```python
from build123d import *

# Parameters (mm, degrees)
SKETCH_1_R          = 3.25
EXTRUDE_1_DEPTH     = 28
SKETCH_3_R          = 4.25
CUT_EXTRUDE_1_DEPTH = 17


with BuildPart() as part:
    # 草图1 → 凸台-拉伸1 (new, symmetric)
    with BuildSketch(Plane.XY):
        with BuildLine():
            Line((-77.585786438, 0), (0, 0))
            Line((0, 0), (0, 8))
            Line((0, 8), (-17.995464086, 8))
            Line((-17.995464086, 8), (-30.499317942, 38.186973559))
            Line((-30.499317942, 38.186973559), (-17.774603256, 50.911688245))
            Line((-17.774603256, 50.911688245), (-23.431457505, 56.568542495))
            Line((-23.431457505, 56.568542495), (-78.292893219, 1.707106781))
            ThreePointArc((-78.292893219, 1.707106781), (-78.50966597, 0.617316568), (-77.585786438, 0))
        make_face()
        with Locations((-57.82689122, 9.184402377)):
            Circle(SKETCH_1_R, mode=Mode.SUBTRACT)
        Polygon((-67.928932188, 5), (-63.07447047, 5), (-64.496309389, 8.4326228), align=None, mode=Mode.SUBTRACT)
        with BuildLine():
            Line((-54.257468753, 5), (-20, 5))
            Line((-20, 5), (-34.038059223, 38.890872965))
            Line((-34.038059223, 38.890872965), (-58.261747684, 14.667184504))
            ThreePointArc((-58.261747684, 14.667184504), (-52.745553791, 11.289161255), (-54.257468753, 5))
        make_face(mode=Mode.SUBTRACT)
    extrude(amount=EXTRUDE_1_DEPTH, both=True)

    # 草图3 → 切除-拉伸1 (cut)
    with BuildSketch(Plane(origin=(0, 8, 0), x_dir=(1, 0, 0), z_dir=(0, 1, 0))):
        with Locations(Location((-10, -15, 0), (0, 0, 180))):
            Circle(SKETCH_3_R)
        with Locations(Location((-10, 15, 0), (0, 0, 270))):
            Circle(SKETCH_3_R)
    cut_extrude_1 = extrude(amount=-CUT_EXTRUDE_1_DEPTH, mode=Mode.SUBTRACT)

    # 镜向1: 切除-拉伸1 across plane
    add(cut_extrude_1.mirror(Plane(origin=(-11.715728753, 28.284271247, 0), x_dir=(0, 0, 1), z_dir=(-0.3826834323650881, 0.9238795325112875, 0))), mode=Mode.SUBTRACT)


solid = part.part
```
Design review of the part built by this model. Coordinates are the model's own, in mm. A direction names the side the tool comes from. Coordinates: 2 decimals unless noted, no trailing zeros. Order: outer loops, then holes, each group sorted by start corner. A loop starts at its lowest first (then second) coordinate and runs counter-clockwise, first axis right, second up. Notation, with made-up numbers: (60, 39) - (98, 39) arc R25 cw to (98, 73) - close; hole circle Ø11 at (8, -7.75). An arc over 180 degrees is marked (long way). Answer in a Markdown table with one row per item.
(1) Consider section C-C on y = 35. State the section outline as (x, z) points.
Checked values:
| item | result |
|---|---|
| outline | (-45, -28) - (-37.93, -28) - (-37.93, 28) - (-45, 28) - close; (-32.43, -28) - (-29.18, -28) - (-29.18, 28) - (-32.43, 28) - close |
(2) For faces 5 (the flat face through (0, 4, 0)), 6 (the flat face through (-63.775, 6.692, 0.392)), list the 3-axis set-ups (+Z, -Z, +X, -X, +Y, -Y) from which the entire face can be reached by the end or side of a thin tool; tool diameter is ignored.
Checked values:
| item | result |
|---|---|
| face 5 | +Z, -Z, +X, +Y, -Y |
| face 6 | +Z, -Z |
(3) The part is to be moulded in two halves that separate along Y. For faces 1 (the flat face through (-45.98, 26.95, 0.39)), 2 (the flat face through (-51.1, 22.1, -28)), 3 (the cylindrical face through (-78.516, 0.633, 0.392)), 4 (the flat face through (-50, 30, 0)), say which applies: released by +Y, released by -Y, zero draft, split by the parting line, or undercut.
Checked values:
| item | result |
|---|---|
| face 1 | undercut |
| face 2 | zero draft |
| face 3 | split by the parting line |
| face 4 | released by +Y |
(4) Clearance check with flat-ended pins moving along their axes: pin 1 (7.5 mm diameter, centred on x = -10, z = 15, fed in from +Y); pin 2 (2.5 mm diameter, centred on x = -65.5, z = 11.5, fed in from +Y); pin 3 (2 mm diameter, centred on x = -51.5, z = -15.5, fed in from +Y); pin 4 (3 mm diameter, centred on x = -47, z = 19, fed in from +Y). State where each tip first meets the part, or that it passes through.
Checked values:
| item | result |
|---|---|
| pin 1 | through |
| pin 2 | y = 15.75 |
| pin 3 | y = 29.5 |
| pin 4 | y = 34.5 |
(5) Wall thickness on line 1 along Y through (x, z) = (-24, 1.5); line 2 along X through (y, z) = (5.5, 4); line 3 along Y through (x, z) = (-16.5, 16.5): over which ranges is each line inside the solid? List them lowest first. Write a range as from..to.
Checked values:
| item | result |
|---|---|
| line 1 | 0..5, 14.66..22.5, 44.69..56 |
| line 2 | -74.5..-67.43, -63.28..-53.74, -20.21..0 |
| line 3 | 0..8 |
(6) Consider section A-A on x = -10. State the section outline as (y, z) points, plus the area to 3 significant figures.
Checked values:
| item | result |
|---|---|
| outline | (0, -28) - (8, -28) - (8, -19.25) - (0, -19.25) - close; (0, -10.75) - (8, -10.75) - (8, 10.75) - (0, 10.75) - close; (0, 19.25) - (8, 19.25) - (8, 28) - (0, 28) - close |
| area | 312 mm^2 |
(7) Consider section D-D on x = -50. State the section outline as (y, z) points.
Checked values:
| item | result |
|---|---|
| outline | (0, -28) - (5, -28) - (5, 28) - (0, 28) - close; (22.93, -28) - (30, -28) - (30, 28) - (22.93, 28) - close |
(8) Consider section B-B on z = 15. State the section outline as (x, y) points, plus the area to 3 significant figures.
Checked values:
| item | result |
|---|---|
| outline | (-78.29, 1.71) arc R1 ccw to (-77.59, 0) - (-14.25, 0) - (-14.25, 8) - (-18, 8) - (-30.5, 38.19) - (-27.85, 40.84) - (-33.51, 46.49) - close; (-27.5, 52.5) - (-21.84, 46.85) - (-17.77, 50.91) - (-23.43, 56.57) - close; (-5.75, 0) - (0, 0) - (0, 8) - (-5.75, 8) - close; hole (-67.93, 5) - (-63.07, 5) - (-64.5, 8.43) - close; hole circle Ø6.5 at (-57.83, 9.18); hole (-58.26, 14.67) arc R5.5 cw to (-54.26, 5) - (-20, 5) - (-34.04, 38.89) - close |
| area | 874 mm^2 |
